```python
from build123d import *

# Parameters (mm, degrees)
SKETCH_1_W          = 42
SKETCH_1_H          = 42
EXTRUDE_1_DEPTH     = 17
SKETCH_2_W          = 42
SKETCH_2_H          = 32.5
CUT_EXTRUDE_1_DEPTH = 12.4
SKETCH_3_R          = 11.05
CUT_EXTRUDE_2_DEPTH = 12.4
SKETCH_4_R          = 2.5
CUT_EXTRUDE_3_DEPTH = 12.4
SKETCH_5_R          = 1.25
CUT_EXTRUDE_4_DEPTH = 12.4
FILLET_1_R          = 3
CHAMFER_1_SIZE      = 0.2
CHAMFER_2_SIZE      = 0.2
CHAMFER_3_SIZE      = 0.2
SKETCH_6_R          = 1.75
CUT_EXTRUDE_5_DEPTH = 26
CHAMFER_4_SIZE      = 0.2


with BuildPart() as part:
    # Эскиз1 → Бобышка-Вытянуть1 (new body)
    with BuildSketch(Plane.XY):
        with Locations((21, 21)):
            Rectangle(SKETCH_1_W, SKETCH_1_H)
    extrude(amount=EXTRUDE_1_DEPTH)

    # Эскиз2 → Вырез-Вытянуть1 (cut)
    with BuildSketch(Plane.XY.offset(17)):
        with Locations((21, 25.75)):
            Rectangle(SKETCH_2_W, SKETCH_2_H)
    extrude(amount=-CUT_EXTRUDE_1_DEPTH, mode=Mode.SUBTRACT)

    # Эскиз3 → Вырез-Вытянуть2 (cut)
    with BuildSketch(Plane(origin=(0, 0, 0), x_dir=(-1, 0, 0), z_dir=(0, 0, -1))):
        with Locations((-21, 21)):
            Circle(SKETCH_3_R)
    extrude(amount=-CUT_EXTRUDE_2_DEPTH, mode=Mode.SUBTRACT)

    # Эскиз4 → Вырез-Вытянуть3 (cut)
    with BuildSketch(Plane(origin=(0, 9.5, 0), x_dir=(1, 0, 0), z_dir=(0, 1, 0))):
        with Locations((15, -12)):
            Circle(SKETCH_4_R)
    extrude(amount=-CUT_EXTRUDE_3_DEPTH, mode=Mode.SUBTRACT)

    # Эскиз5 → Вырез-Вытянуть4 (cut)
    with BuildSketch(Plane(origin=(0, 9.5, 0), x_dir=(1, 0, 0), z_dir=(0, 1, 0))):
        with Locations((32, -10)):
            Circle(SKETCH_5_R)
    extrude(amount=-CUT_EXTRUDE_4_DEPTH, mode=Mode.SUBTRACT)

    # Скругление1
    fillet_1_edges = [part.edges().sort_by_distance(p)[0] for p in [
        (0, 42, 2.3),
        (42, 42, 2.3),
        (0, 9.5, 10.8),
        (42, 9.5, 10.8),
        (42, 0, 8.5),
        (0, 0, 8.5),
    ]]
    fillet(fillet_1_edges, radius=FILLET_1_R)

    # Фаска1
    chamfer_1_edges = [part.edges().sort_by_distance(p)[0] for p in [
        (32.05, 21, 0),
        (21, 42, 0),
        (0, 21, 0),
        (42, 21, 0),
        (21, 0, 0),
        (0.878679656, 0.878679656, 0),
        (41.121320344, 0.878679656, 0),
        (0.878679656, 41.121320344, 0),
        (41.121320344, 41.121320344, 0),
    ]]
    chamfer(chamfer_1_edges, length=CHAMFER_1_SIZE)

    # Фаска2
    chamfer_2_edges = [part.edges().sort_by_distance(p)[0] for p in [
        (42, 24.25, 4.6),
        (21, 42, 4.6),
        (42, 4.75, 17),
        (0, 24.25, 4.6),
        (0.878679656, 41.121320344, 4.6),
        (41.121320344, 41.121320344, 4.6),
        (0, 4.75, 17),
        (21, 0, 17),
        (21, 9.5, 17),
        (0.878679656, 8.621320344, 17),
        (0.878679656, 0.878679656, 17),
        (41.121320344, 8.621320344, 17),
        (41.121320344, 0.878679656, 17),
    ]]
    chamfer(chamfer_2_edges, length=CHAMFER_2_SIZE)

    # Фаска3
    chamfer_3_edges = [part.edges().sort_by_distance(p)[0] for p in [
        (32.05, 21, 4.6),
    ]]
    chamfer(chamfer_3_edges, length=CHAMFER_3_SIZE)

    # Эскиз6 → Вырез-Вытянуть5 (cut)
    with BuildSketch(Plane(origin=(0, 0, 0), x_dir=(-1, 0, 0), z_dir=(0, 0, -1))):
        with Locations((-5.5, 36.5)):
            Circle(SKETCH_6_R)
        with Locations((-36.5, 36.5)):
            Circle(SKETCH_6_R)
        with Locations((-5.5, 5.5)):
            Circle(SKETCH_6_R)
        with Locations((-36.5, 5.5)):
            Circle(SKETCH_6_R)
    extrude(amount=-CUT_EXTRUDE_5_DEPTH, mode=Mode.SUBTRACT)

    # Фаска4
    chamfer_4_edges = [part.edges().sort_by_distance(p)[0] for p in [
        (7.25, 36.5, 4.6),
        (7.25, 36.5, 0),
        (38.25, 36.5, 4.6),
        (38.25, 36.5, 0),
        (7.25, 5.5, 17),
        (7.25, 5.5, 0),
        (38.25, 5.5, 17),
        (38.25, 5.5, 0),
    ]]
    chamfer(chamfer_4_edges, length=CHAMFER_4_SIZE)


solid = part.part
```
Model file for the job. Use its own axes, mm. A direction names the side the tool comes from. Coordinates: 2 decimals unless noted, no trailing zeros. Order: outer loops, then holes, each group sorted by start corner. A loop starts at its lowest first (then second) coordinate and runs counter-clockwise, first axis right, second up. Notation, with made-up numbers: (34.5, -2) -> (66.5, -2) arc R10 ccw to (66.5, 17) -> close; hole circle Ø8 at (13, 8.25). An arc over 180 degrees is marked (long way). Answer as a JSON object with one key per item and string values. Group by question number.
1) Cut at C-C, the plane x = 36.5. Write the cut outline in (y, z), then the cut area to 3 significant figures.
2) Cut at B-B, the plane y = 36.5. Write the cut outline in (x, z), then the cut area to 3 significant figures.
3) Drill centre lines: L1, parallel to Y at x = 36.5, z = 3.45; L2, parallel to X at y = 4.5, z = 10; L3, parallel to Z at x = 25.5, y = 34. Where is each one in solid material? Low to high.
4) Cut at D-D, the plane y = 5.5. Write the cut outline in (x, z).
5) Flat gauge pins, fed straight in: pin 1 (2 mm diameter, centred on x = 32.5, y = 32.5, fed in from +Z); pin 2 (1 mm diameter, centred on x = 10.5, y = 21, fed in from +Z); pin 3 (10 mm diameter, centred on x = 24, z = 10, fed in from +Y). Where does each tip first touch, or does it go through?
6) Cut at A-A, the plane z = 12. Write the cut outline in (x, y), then the cut area to 3 significant figures.
7) Which spindle directions (+Z, -Z, +X, -X, +Y, -Y) get a long thin tool onto all of the face, cutting with end or side? Do faces 1 (the face through (41.1, 8.64, 10.51)), 2 (the face through (21, 9.5, 11)), 3 (the face through (42, 17, 4)). Say none if no direction does.
Check values:
{
 "1": {"outline": "(0, 0.2) -> (0.2, 0) -> (3.55, 0) -> (3.75, 0.2) -> (3.75, 16.8) -> (3.55, 17) -> (0.2, 17) -> (0, 16.8) -> close; (7.25, 0.2) -> (7.45, 0) -> (34.55, 0) -> (34.75, 0.2) -> (34.75, 4.4) -> (34.55, 4.6) -> (9.5, 4.6) -> (9.5, 16.8) -> (9.3, 17) -> (7.45, 17) -> (7.25, 16.8) -> close; (38.25, 0.2) -> (38.45, 0) -> (41.8, 0) -> (42, 0.2) -> (42, 4.4) -> (41.8, 4.6) -> (38.45, 4.6) -> (38.25, 4.4) -> close", "area": "235 mm²"},
 "2": {"outline": "(0, 0.2) -> (0.2, 0) -> (3.55, 0) -> (3.75, 0.2) -> (3.75, 4.4) -> (3.55, 4.6) -> (0.2, 4.6) -> (0, 4.4) -> close; (7.25, 0.2) -> (7.45, 0) -> (34.55, 0) -> (34.75, 0.2) -> (34.75, 4.4) -> (34.55, 4.6) -> (7.45, 4.6) -> (7.25, 4.4) -> close; (38.25, 0.2) -> (38.45, 0) -> (41.8, 0) -> (42, 0.2) -> (42, 4.4) -> (41.8, 4.6) -> (38.45, 4.6) -> (38.25, 4.4) -> close", "area": "161 mm²"},
 "3": {"L1": "y = 0 to 3.75, 7.25 to 34.75, 38.25 to 42", "L2": "x = 0 to 4.06, 6.94 to 13.5, 16.5 to 30.75, 33.25 to 35.06, 37.94 to 42", "L3": "z = 0 to 4.6"},
 "4": {"outline": "(0, 0.2) -> (0.2, 0) -> (3.55, 0) -> (3.75, 0.2) -> (3.75, 16.8) -> (3.55, 17) -> (0.2, 17) -> (0, 16.8) -> close; (7.25, 0.2) -> (7.45, 0) -> (34.55, 0) -> (34.75, 0.2) -> (34.75, 16.8) -> (34.55, 17) -> (7.45, 17) -> (7.25, 16.8) -> close; (38.25, 0.2) -> (38.45, 0) -> (41.8, 0) -> (42, 0.2) -> (42, 16.8) -> (41.8, 17) -> (38.45, 17) -> (38.25, 16.8) -> close; hole circle Ø5 at (15, 12); hole circle Ø2.5 at (32, 10)"},
 "5": {"pin 1": "stops at z = 4.6", "pin 2": "passes through", "pin 3": "stops at y = 9.5"},
 "6": {"outline": "(0, 3) arc R3 ccw to (3, 0) -> (12.5, 0) -> (12.5, 9.5) -> (3, 9.5) arc R3 ccw to (0, 6.5) -> close; (17.5, 0) -> (39, 0) arc R3 ccw to (42, 3) -> (42, 6.5) arc R3 ccw to (39, 9.5) -> (17.5, 9.5) -> close; hole circle Ø3.5 at (5.5, 5.5); hole circle Ø3.5 at (36.5, 5.5)", "area": "325 mm²"},
 "7": {"face 1": "+Z, +X, +Y", "face 2": "+Z, +X, -X, +Y", "face 3": "+Z, -Z, +X, +Y, -Y"}
}
